Here's how the part is built. I have some questions about the finished solid (model axes, mm). Face numbers are marked on the shaded views. A direction names the side the tool comes from. Coordinates: 2 decimals unless noted, no trailing zeros. Order: outer loops, then holes, each group sorted by start corner. A loop starts at its lowest first (then second) coordinate and runs counter-clockwise, first axis right, second up. Notation, with made-up numbers: (88, 63.25) - (114, 63.25) arc R32 cw to (114, 102.25) - close; hole circle Ø1 at (19, -9.5). An arc over 180 degrees is marked (long way). Answer as CSV lines item,"result". Start each with the question number.
Item 1: Imagine slicing it at D-D on y = 11. List the corners of the cut face in (x, z) for me, and give its area (3 significant figures).
Item 2: Imagine slicing it at A-A on y = 0. List the corners of the cut face in (x, z) for me.
Item 3: I'm going to push a flat-ended pin straight in: pin 1 (8 mm diameter, centred on y = -1, z = 1, fed in from -X). Where does the tip first touch, or does it pass through?
Item 4: Imagine slicing it at C-C on x = 1.55. List the corners of the cut face in (y, z) for me.
Item 5: Imagine slicing it at B-B on z = 0. List the corners of the cut face in (x, y) for me, and give its area (3 significant figures).
Item 6: I need wall thicknesses on line 1 (Y direction, x = 0.7, z = -29.5); line 2 (Z direction, x = 1.6, y = 1.25); line 3 (Z direction, x = 0.15, y = 11). Which ranges of each line are inside material? Lowest first, please.
Item 7: On a 3-axis mill with a long thin cutter (end or side, diameter ignored), from which of +Z, -Z, +X, -X, +Y, -Y can I reach the whole of each face in a straight line? I mean the marked faces 1 and 2. Say none if no direction works.
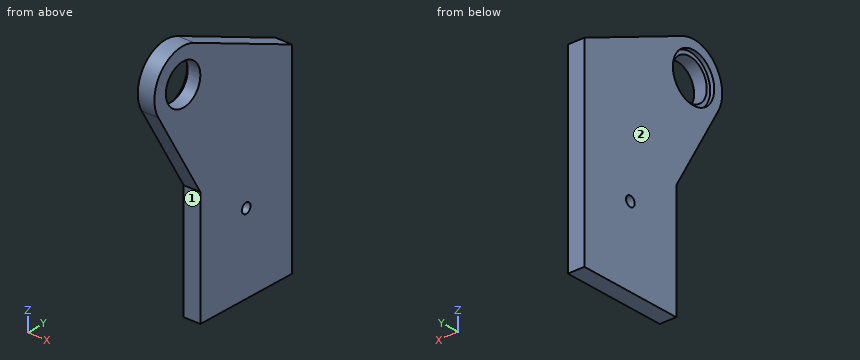
Autodesk Inventor part; units mm, degrees
ref_plane "YZ Plane" through (0, 0, 0) normal (1, 0, 0) x (0, 1, 0)
ref_plane "XZ Plane" through (0, 0, 0) normal (0, 1, 0) x (-1, 0, 0)
ref_plane "XY Plane" through (0, 0, 0) normal (0, 0, 1) x (1, 0, 0)
sketch "スケッチ1" plane through (0, 0, 0) normal (1, 0, 0) x (0, 1, 0)
  circle A0 centre (0, 0) radius 5 construction
  circle A1 centre (0, 0) radius 3.6
  arc A2 (1.9342, 4.6107) -> (-4.3208, -2.5162) centre (0, 0) ccw
  line L0 (-4.3208, -2.5162) -> (3, -15.0874)
  line L1 (3, -15.0874) -> (3, -32.1321)
  line L2 (3, -32.1321) -> (19, -32.1321)
  line L3 (19, -32.1321) -> (19, -2.5484)
  line L4 (19, -2.5484) -> (1.9342, 4.6107)
  circle A3 centre (0, 0) radius 3
  circle A4 centre (11, -20.4215) radius 0.75
  circle A5 centre (11, -20.4215) radius 5 construction
  circle A6 centre (16, -20.4215) radius 1 construction
  line L5 (16, -20.4215) -> (6, -20.4215) construction
  circle A7 centre (6, -20.4215) radius 1 construction
  circle A8 centre (11, -20.4215) radius 8 construction
  dimension "d1" = 10
  dimension "d0" = 7.2
  dimension "d4" = 6
  dimension "d7" = 1.5
  dimension "d8" = 10
  dimension "d9" = 2
  dimension "d11" = 16
extrude "押し出し1" add sketch "スケッチ1" along normal blind 2.5 contours A1 | L4 L3 L2 L1 L0 A2
extrude "押し出し2" cut sketch "スケッチ1" along normal blind 0.6 contours A1 | A3
properties part number "Gear_Frame"
Responses:
1,outline,"(0, -32.13) - (2.5, -32.13) - (2.5, -21.17) - (0, -21.17) - close; (0, -19.67) - (2.5, -19.67) - (2.5, 0.81) - (0, 0.81) - close"
1,area,"78.6 mm^2"
2,outline,"(0, -9.94) - (2.5, -9.94) - (2.5, -3) - (0.6, -3) - (0.6, -3.6) - (0, -3.6) - close; (0, 3.6) - (0.6, 3.6) - (0.6, 3) - (2.5, 3) - (2.5, 5) - (0, 5) - close"
3,pin 1,"stops at x = 0"
4,outline,"(-4.32, -2.52) - (3, -15.09) - (3, -32.13) - (19, -32.13) - (19, -2.55) - (1.93, 4.61) arc R5 ccw to start; hole circle Ø6 at (0, 0); hole circle Ø1.5 at (11, -20.42)"
5,outline,"(0, -5) - (2.5, -5) - (2.5, -3) - (0.6, -3) - (0.6, -3.6) - (0, -3.6) - close; (0, 3.6) - (0.6, 3.6) - (0.6, 3) - (2.5, 3) - (2.5, 12.93) - (0, 12.93) - close"
5,area,"29.1 mm^2"
6,line 1,"y = 3 to 19"
6,line 2,"z = -12.08 to -2.73, 2.73 to 4.84"
6,line 3,"z = -32.13 to -21.17, -19.67 to 0.81"
7,face 1,"-Z, +X, -X, -Y"
7,face 2,"+Z, -Z, -X, +Y, -Y"
